Can you work these out from the model? Positions are in its coordinate system, mm. A direction names the side the tool comes from. Give positions to 0.01 mm unless a question says otherwise; leave off trailing zeros. Write each loop counter-clockwise with the first axis right and the second up, starting at its lowest first coordinate (ties: lowest second). Pieces come first, ordered by that corner, then holes.
1. If I drill on probe 1 along Y at (x, z) = (-4, -9); probe 2 along Z at (x, y) = (7.25, 0.45); probe 3 along X at (y, z) = (2.4, 11.5), over which ranges is the centre line in solid material (lowest first)?
2. Suppose I cut it at A-A (y = 3.8). Please give me the cut outline in (x, z), and give its area (3 significant figures).
3. Suppose I cut it at B-B (z = 5.5). Please give me the cut outline in (x, y).
4. I'm going to push flat-ended pins straight in: pin 1 (3 mm diameter, centred on x = -5, y = 1.5, fed in from +Z); pin 2 (1 mm diameter, centred on y = 2.5, z = 13, fed in from -X); pin 3 (1.6 mm diameter, centred on x = 5.5, y = 3, fed in from -Z). Where does each tip first touch, or does it pass through?
5. Suppose I cut it at C-C (y = 1.4). Please give me the cut outline in (x, z), and give its area (3 significant figures).
6. On a 3-axis mill with a long thin cutter (end or side, diameter ignored), from which of +Z, -Z, +X, -X, +Y, -Y can I reach the whole of each face in a straight line? I mean faces 1 (the flat face through (-2.25, 3, 13)), 2 (the flat face through (-5, 3, -11.05)), 3 (the flat face through (2.25, 3, -13)). Say none if no direction works.
7. Thinking about a two-plate mould opening in Z: for faces 4 (the flat face through (5, 3, -11.05)), 5 (the flat face through (0, 0, 0)), 6 (the cylindrical face through (0, 4, 10)), which applies, pulls with the +Z half, pulls with the -Z half, needs draft (parallel to the pull), parting line crosses it, or undercut?
8. Suppose I cut it at D-D (x = 5.75). Please give me the cut outline in (y, z), and give its area (3 significant figures).
```python
from build123d import *

# Parameters (mm, degrees)
SKETCH1_W           = 5.75
SKETCH1_H           = 22.1
SKETCH1_W_2         = 4.5
SKETCH1_H_2         = 3.2
BOSS_EXTRUDE1_DEPTH = 5.5
SKETCH2_R           = 10
CUT_EXTRUDE1_DEPTH  = 3.2
CHAMFER1_SIZE       = 1
SKETCH3_W           = 3.5
SKETCH3_H           = 31
BOSS_EXTRUDE2_DEPTH = 0.25


with BuildPart() as part:
    # Sketch1 → Boss-Extrude1 (new body)
    with BuildSketch(Plane(origin=(0, 0, 0), x_dir=(1, 0, 0), z_dir=(0, 1, 0))):
        with Locations((-5.125, 0)):
            Rectangle(SKETCH1_W, SKETCH1_H)
        Rectangle(SKETCH1_W_2, SKETCH1_H)
        with Locations((0, 12.65)):
            Rectangle(SKETCH1_W_2, SKETCH1_H_2)
        with Locations((0, -12.65)):
            Rectangle(SKETCH1_W_2, SKETCH1_H_2)
        with Locations((5.125, 0)):
            Rectangle(SKETCH1_W, SKETCH1_H)
    extrude(amount=BOSS_EXTRUDE1_DEPTH)

    # Sketch2 → Cut-Extrude1 (cut)
    with BuildSketch(Plane(origin=(0, 5.5, 0), x_dir=(1, 0, 0), z_dir=(0, 1, 0))):
        Circle(SKETCH2_R)
    extrude(amount=-CUT_EXTRUDE1_DEPTH, mode=Mode.SUBTRACT)

    # Chamfer1
    chamfer1_edges = [part.edges().sort_by_distance(p)[0] for p in [
        (-8, 2.75, -11.05),
    ]]
    chamfer(chamfer1_edges, length=CHAMFER1_SIZE)

    # Sketch3 → Boss-Extrude2 (add)
    with BuildSketch(Plane.XZ):
        Rectangle(SKETCH3_W, SKETCH3_H)
    extrude(amount=-BOSS_EXTRUDE2_DEPTH)


solid = part.part
```
Checks:
1. probe 1: y = 0 to 2.3
1. probe 2: z = -11.05 to 11.05
1. probe 3: x = -2.25 to 2.25
2. outline: (-8, -10.05) - (-7, -11.05) - (-2.25, -11.05) - (-2.25, -14.25) - (2.25, -14.25) - (2.25, -11.05) - (8, -11.05) - (8, -6) arc R10 cw to (-8, -6) - close; (-8, 6) arc R10 cw to (8, 6) - (8, 11.05) - (2.25, 11.05) - (2.25, 14.25) - (-2.25, 14.25) - (-2.25, 11.05) - (-8, 11.05) - close
2. area: 100 mm2
3. outline: (-8, 0) - (8, 0) - (8, 2.3) - (-8, 2.3) - close
4. pin 1: stops at z = 11.05
4. pin 2: stops at x = -2.25
4. pin 3: stops at z = -11.05
5. outline: (-8, -10.05) - (-7, -11.05) - (-2.25, -11.05) - (-2.25, -14.25) - (2.25, -14.25) - (2.25, -11.05) - (8, -11.05) - (8, 11.05) - (2.25, 11.05) - (2.25, 14.25) - (-2.25, 14.25) - (-2.25, 11.05) - (-8, 11.05) - close
5. area: 382 mm2
6. face 1: +Z, -X, +Y, -Y
6. face 2: -Z, -X, +Y, -Y
6. face 3: -Z, +X, +Y, -Y
7. face 4: pulls with the -Z half
7. face 5: needs draft
7. face 6: undercut
8. outline: (0, -11.05) - (5.5, -11.05) - (5.5, -8.18) - (2.3, -8.18) - (2.3, 8.18) - (5.5, 8.18) - (5.5, 11.05) - (0, 11.05) - close
8. area: 69.2 mm2
